from build123d import *

# Parameters (mm, degrees)
BOSS_EXTRU_1_DEPTH  = 300
SYM_TRIE6_OUTLINE_R = 2.1
SYM_TRIE6_DEPTH     = 300


# Read off the part's stored shape, not the designer's step: Symétrie6
with BuildPart() as part:
    # Esquisse1 → Boss.-Extru.1 (new body)
    with BuildSketch(Plane.XY):
        with BuildLine():
            Line((-9.5, 10), (-4.58, 10))
            Line((-4.58, 10), (-3.125, 8.545))
            Line((-3.125, 8.545), (-3.125, 8.2))
            Line((-3.125, 8.2), (-5.5, 8.2))
            Line((-5.5, 8.2), (-5.5, 6.560660172))
            Line((-5.5, 6.560660172), (-2.839339828, 3.9))
            Line((-2.839339828, 3.9), (-0.21, 3.9))
            Line((-0.21, 3.9), (0, 3.69))
            Line((0, 3.69), (0, 2.1))
            ThreePointArc((0, 2.1), (-2.1, 0), (0, -2.1))
            Line((0, -2.1), (0, -3.69))
            Line((0, -3.69), (-0.21, -3.9))
            Line((-0.21, -3.9), (-2.839339828, -3.9))
            Line((-2.839339828, -3.9), (-6.239339828, -7.3))
            Line((-6.239339828, -7.3), (-8.2, -7.3))
            Line((-8.2, -7.3), (-8.2, -10))
            Line((-8.2, -10), (-10, -10))
            Line((-10, -10), (-10, -4.58))
            Line((-10, -4.58), (-8.545, -3.125))
            Line((-8.545, -3.125), (-8.2, -3.125))
            Line((-8.2, -3.125), (-8.2, -5.5))
            Line((-8.2, -5.5), (-6.560660172, -5.5))
            Line((-6.560660172, -5.5), (-3.9, -2.839339828))
            Line((-3.9, -2.839339828), (-3.9, -0.21))
            Line((-3.9, -0.21), (-3.69, 0))
            Line((-3.69, 0), (-3.9, 0.21))
            Line((-3.9, 0.21), (-3.9, 2.839339828))
            Line((-3.9, 2.839339828), (-6.560660172, 5.5))
            Line((-6.560660172, 5.5), (-8.2, 5.5))
            Line((-8.2, 5.5), (-8.2, 3.125))
            Line((-8.2, 3.125), (-8.545, 3.125))
            Line((-8.545, 3.125), (-10, 4.58))
            Line((-10, 4.58), (-10, 9.5))
            ThreePointArc((-10, 9.5), (-9.853553391, 9.853553391), (-9.5, 10))
        make_face()
    boss_extru_1 = extrude(amount=BOSS_EXTRU_1_DEPTH)

    # Symétrie1: Boss.-Extru.1 across Right Plane
    add(boss_extru_1.mirror(Plane(origin=(0, 0, 0), x_dir=(0, 0, -1), z_dir=(1, 0, 0))))

    # Symétrie6 outline → Symétrie6 (add)
    with BuildSketch(Plane.XY):
        with BuildLine():
            Line((-3.9, -17.160660172), (-3.9, -19.79))
            Line((-3.9, -19.79), (-3.69, -20))
            Line((-3.69, -20), (-3.9, -20.21))
            Line((-3.9, -20.21), (-3.9, -22.839339828))
            Line((-3.9, -22.839339828), (-6.560660172, -25.5))
            Line((-6.560660172, -25.5), (-8.2, -25.5))
            Line((-8.2, -25.5), (-8.2, -23.125))
            Line((-8.2, -23.125), (-8.545, -23.125))
            Line((-8.545, -23.125), (-10, -24.58))
            Line((-10, -24.58), (-10, -29.5))
            ThreePointArc((-10, -29.5), (-9.853553391, -29.853553391), (-9.5, -30))
            Line((-9.5, -30), (-4.58, -30))
            Line((-4.58, -30), (-3.125, -28.545))
            Line((-3.125, -28.545), (-3.125, -28.2))
            Line((-3.125, -28.2), (-5.5, -28.2))
            Line((-5.5, -28.2), (-5.5, -26.560660172))
            Line((-5.5, -26.560660172), (-2.839339828, -23.9))
            Line((-2.839339828, -23.9), (-0.21, -23.9))
            Line((-0.21, -23.9), (0, -23.69))
            Line((0, -23.69), (0.21, -23.9))
            Line((0.21, -23.9), (2.839339828, -23.9))
            Line((2.839339828, -23.9), (5.5, -26.560660172))
            Line((5.5, -26.560660172), (5.5, -28.2))
            Line((5.5, -28.2), (3.125, -28.2))
            Line((3.125, -28.2), (3.125, -28.545))
            Line((3.125, -28.545), (4.58, -30))
            Line((4.58, -30), (9.5, -30))
            ThreePointArc((9.5, -30), (9.853553391, -29.853553391), (10, -29.5))
            Line((10, -29.5), (10, -24.58))
            Line((10, -24.58), (8.545, -23.125))
            Line((8.545, -23.125), (8.2, -23.125))
            Line((8.2, -23.125), (8.2, -25.5))
            Line((8.2, -25.5), (6.560660172, -25.5))
            Line((6.560660172, -25.5), (3.9, -22.839339828))
            Line((3.9, -22.839339828), (3.9, -20.21))
            Line((3.9, -20.21), (3.69, -20))
            Line((3.69, -20), (3.9, -19.79))
            Line((3.9, -19.79), (3.9, -17.160660172))
            Line((3.9, -17.160660172), (6.560660172, -14.5))
            Line((6.560660172, -14.5), (8.2, -14.5))
            Line((8.2, -14.5), (8.2, -16.875))
            Line((8.2, -16.875), (8.545, -16.875))
            Line((8.545, -16.875), (10, -15.42))
            Line((10, -15.42), (10, -10))
            Line((10, -10), (8.2, -10))
            Line((8.2, -10), (8.2, -12.7))
            Line((8.2, -12.7), (6.239339828, -12.7))
            Line((6.239339828, -12.7), (2.839339828, -16.1))
            Line((2.839339828, -16.1), (0.21, -16.1))
            Line((0.21, -16.1), (0, -16.31))
            Line((0, -16.31), (-0.21, -16.1))
            Line((-0.21, -16.1), (-2.839339828, -16.1))
            Line((-2.839339828, -16.1), (-6.239339828, -12.7))
            Line((-6.239339828, -12.7), (-8.2, -12.7))
            Line((-8.2, -12.7), (-8.2, -10))
            Line((-8.2, -10), (-10, -10))
            Line((-10, -10), (-10, -15.42))
            Line((-10, -15.42), (-8.545, -16.875))
            Line((-8.545, -16.875), (-8.2, -16.875))
            Line((-8.2, -16.875), (-8.2, -14.5))
            Line((-8.2, -14.5), (-6.560660172, -14.5))
            Line((-6.560660172, -14.5), (-3.9, -17.160660172))
        make_face()
        with Locations((0, -20)):
            Circle(SYM_TRIE6_OUTLINE_R, mode=Mode.SUBTRACT)
    extrude(amount=SYM_TRIE6_DEPTH)


solid = part.part
Verification items for the finished model (mm, model axes). A direction names the side the tool comes from. Give positions to 0.01 mm unless a question says otherwise; leave off trailing zeros. Write each question's results on one line, items separated by ' | '.
1) Tool access check on faces 1 (the flat face through (8.2, -10, 148)), 2 (the flat face through (-5, -5, 300)). Record the directions out of +Z, -Z, +X, -X, +Y, -Y that give a thin tool (end or side, any length) a straight path to the whole face; none if there is none.
Solution:
face 1: +Z, -Z | face 2: +Z, +X, -X, +Y, -Y
2) Sectioned sample at A-A on z = 266.5. Count the separate pieces of the cut face and the enclosed holes in it, plus the area to 3 significant figures.
Solution:
separate pieces: 1 | enclosed holes: 3 | area: 300 mm2
3) Depth check by flat-ended pin: P1, Ø0.8, axis at x = -2, z = 154, coming from the -Y side; P2, Ø0.8, axis at y = -1.5, z = 142, coming from the +X side; P3, Ø0.8, axis at x = 1.5, z = 80, coming from the +Y side. Enter the tip coordinate at first touch or a pass-through.
Solution:
P1: y = -23.9 | P2: x = 3.9 | P3: y = 3.9
4) Material ranges on L1, parallel to Y at x = -7.75, z = 280.5; L2, parallel to Y at x = 0, z = 170.5; L3, parallel to X at y = 4.5, z = 100, recorded low to high. Write a range as from..to.
Solution:
L1: -30..-25.5, -14.5..-12.7, -7.3..-5.5, 5.5..10 | L2: -23.69..-22.1, -17.9..-16.31, -3.69..-2.1, 2.1..3.69 | L3: -9.92..-8.2, -5.56..-3.44, 3.44..5.56, 8.2..9.92
